Geometry: final body of the model. Coordinates: model frame, mm. Give positions to 0.01 mm unless a question says otherwise; leave off trailing zeros. Order: outer loops, then holes, each group sorted by start corner. A loop starts at its lowest first (then second) coordinate and runs counter-clockwise, first axis right, second up. Notation, with made-up numbers: (89, 50) - (125, 50) arc R32 cw to (125, 81) - close; hole circle Ø11 at (66.25, 43). An arc over 180 degrees is marked (long way). Use one line per item in the form item = value.
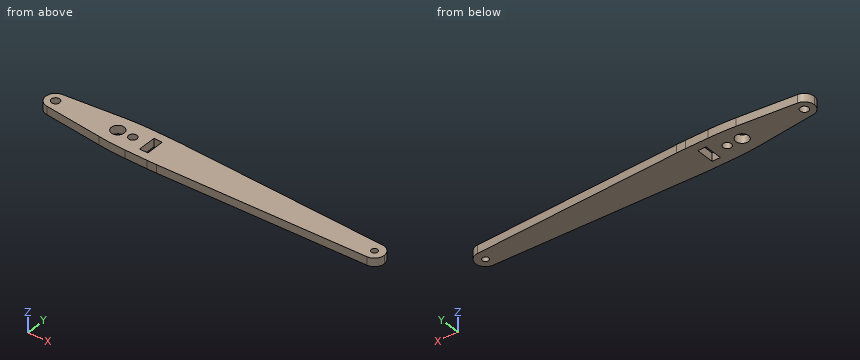
from build123d import *

# Parameters (mm, degrees)
F2_DEPTH = 6.35
F3_R     = 3.175
F3_R_2   = 4.9403
F3_R_3   = 2.413
F4_DEPTH = 6.35
F5_W     = 6.35
F5_H     = 13.97
F6_DEPTH = 6.35


with BuildPart() as f2:
    # F1 (on Top) → F2 (new body)
    with BuildSketch(Plane.XY):
        with BuildLine():
            Line((38.1, 13.212064), (20.927279, 13.212064))
            ThreePointArc((20.927279, 13.212064), (10.449702, 12.941757), (0, 12.131556))
            Line((0, 12.131556), (-43.964773, 7.579481))
            ThreePointArc((-43.964773, 7.579481), (-48.838815, 5.103157), (-50.8, 0))
            ThreePointArc((-50.8, 0), (-48.838815, -5.103157), (-43.964773, -7.579481))
            Line((-43.964773, -7.579481), (0, -12.131556))
            ThreePointArc((0, -12.131556), (10.449702, -12.941757), (20.927279, -13.212064))
            Line((20.927279, -13.212064), (38.1, -13.212064))
            ThreePointArc((38.1, -13.212064), (41.611629, -13.181718), (45.12221, -13.090691))
            Line((45.12221, -13.090691), (203.463333, -7.615448))
            ThreePointArc((203.463333, -7.615448), (208.680465, -5.294233), (210.82, 0))
            ThreePointArc((210.82, 0), (208.680465, 5.294233), (203.463333, 7.615448))
            Line((203.463333, 7.615448), (45.12221, 13.090691))
            ThreePointArc((45.12221, 13.090691), (41.611629, 13.181718), (38.1, 13.212064))
        make_face()
    extrude(amount=-F2_DEPTH)

    # F3 (on face) → F4 (cut, through all)
    with BuildSketch(Plane.XY):
        with Locations((-43.18, 0)):
            Circle(F3_R)
        with Locations((16.51, 0)):
            Circle(F3_R)
        with Locations((4.9276, 0)):
            Circle(F3_R_2)
        with Locations((203.2, 0)):
            Circle(F3_R_3)
    extrude(amount=-F4_DEPTH, mode=Mode.SUBTRACT)

    # F5 (on face) → F6 (cut, through all)
    with BuildSketch(Plane.XY):
        with Locations((30.48, 0)):
            Rectangle(F5_W, F5_H)
    extrude(amount=-F6_DEPTH, mode=Mode.SUBTRACT)


solid = f2.part
(1) Cut plane B-B on x = 16.51. Output: boundary loops of the cut face in (y, z) (3 decimals).
Computed values:
outline = (-13.164, -6.35) - (-3.175, -6.35) - (-3.175, 0) - (-13.164, 0) - close; (3.175, -6.35) - (13.164, -6.35) - (13.164, 0) - (3.175, 0) - close
(2) Cut plane A-A on z = -1.75. Output: boundary loops of the cut face in (x, y) (3 decimals), plus the area to 3 significant figures.
Computed values:
outline = (-43.965, -7.579) - (0, -12.132) arc R203.2 ccw to (20.927, -13.212) - (38.1, -13.212) arc R203.204 ccw to (45.122, -13.091) - (203.463, -7.615) arc R7.62 ccw to (203.463, 7.615) - (45.122, 13.091) arc R203.204 ccw to (38.1, 13.212) - (20.927, 13.212) arc R203.2 ccw to (0, 12.132) - (-43.965, 7.579) arc R7.62 ccw to start; hole circle Ø6.35 at (-43.18, 0); hole circle Ø9.881 at (4.928, 0); hole circle Ø6.35 at (16.51, 0); hole (27.305, -6.985) - (33.655, -6.985) - (33.655, 6.985) - (27.305, 6.985) - close; hole circle Ø4.826 at (203.2, 0)
area = 5,240 mm²
(3) Contact query for flat-ended pins moving along their axis: pin 1 Ø5.5 at (x, y) = (203.2, 0) entering from +Z; pin 2 Ø1.9 at (y, z) = (2.5, -2) entering from -X; pin 3 Ø2 at (x, z) = (145, -3.5) entering from +Y; pin 4 Ø2 at (x, z) = (122.5, -3) entering from -Y. Output: stop coordinate, or through.
Computed values:
pin_1 = 0
pin_2 = -50.64
pin_3 = 9.67
pin_4 = -10.45
(4) Cut plane C-C on x = 166. Output: boundary loops of the cut face in (y, z).
Computed values:
outline = (-8.91, -6.35) - (8.91, -6.35) - (8.91, 0) - (-8.91, 0) - close
(5) Cut plane D-D on x = -19. Output: boundary loops of the cut face in (y, z), plus the area to 3 significant figures.
Computed values:
outline = (-10.16, -6.35) - (10.16, -6.35) - (10.16, 0) - (-10.16, 0) - close
area = 129 mm²
(6) Ray query, line 1 along Y through (x, z) = (-43.18, -5) (3 decimals); line 2 along Y through (x, z) = (203.2, -1.5); line 3 along X through (y, z) = (-0.75, -1.5) (3 decimals). Return the intervals inside material, ascending.
Computed values:
line_1 = -7.661 to -3.175, 3.175 to 7.661
line_2 = -7.62 to -2.41, 2.41 to 7.62
line_3 = -50.763 to -46.265, -40.095 to 0.045, 9.811 to 13.425, 19.595 to 27.305, 33.655 to 200.907, 205.493 to 210.783
